Source: three-view drawing plus pictorial views. Frame: mm from the lowest corner of the part. A direction names the side the tool comes from. Coordinates: 2 decimals unless noted, no trailing zeros. Order: outer loops, then holes, each group sorted by start corner. A loop starts at its lowest first (then second) coordinate and runs counter-clockwise, first axis right, second up. Notation, with made-up numbers: (-2.5, 27.5) - (9.5, 27.5) arc R9 cw to (9.5, 31.5) - close; hole circle Ø4 at (-1, 20). An arc over 180 degrees is marked (long way). One line per question, with ' | ' between items.
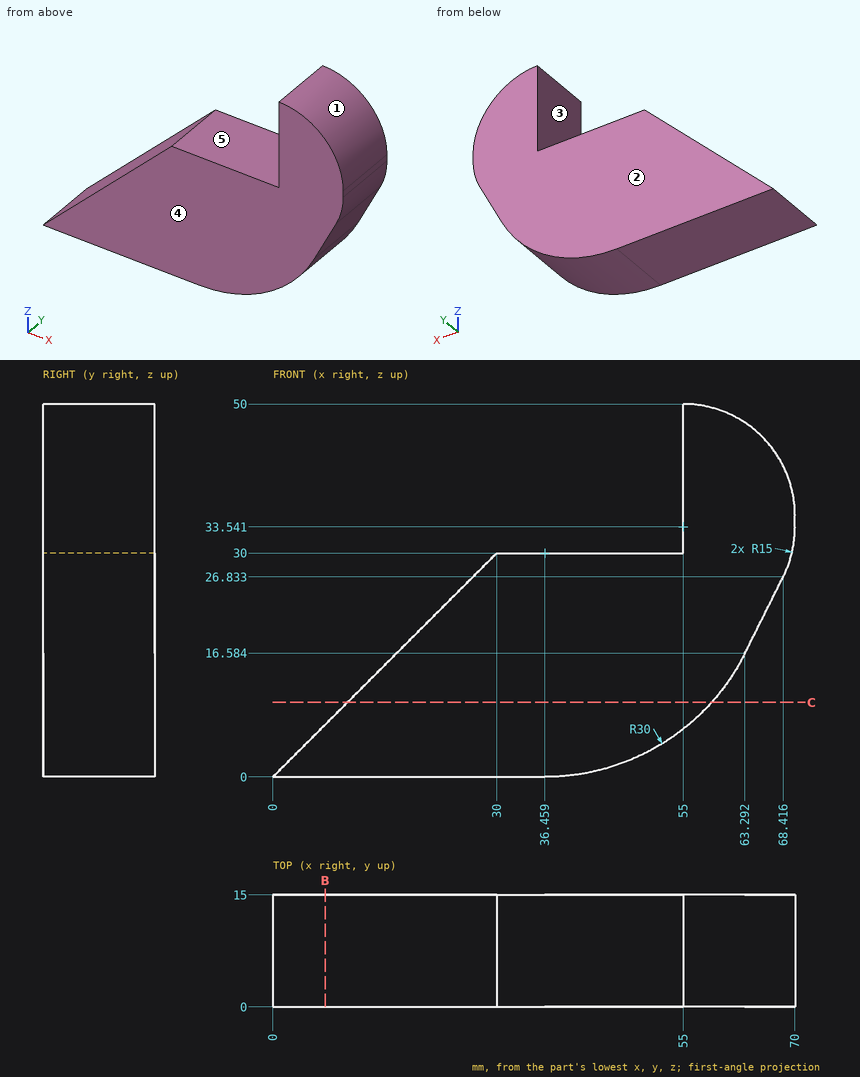
(1) Material intervals for L1, parallel to Z at x = 32, y = 11; L2, parallel to X at y = 4.75, z = 47.5; L3, parallel to X at y = 3, z = 28, sorted ascending. Write a range as from..to.
Taken from the geometry:
L1: z = 0..30 | L2: x = 55..63.29 | L3: x = 28..68.94
(2) Pin query (flat end, axial travel): P1, Ø2, axis at x = 57.5, y = 3.5, coming from the -Z side (1 decimal); P2, Ø8, axis at x = 21.5, y = 4.5, coming from the +Z side; P3, Ø1.5, axis at y = 5, z = 37, coming from the -X side. Return the tip coordinate at first contact, or that it passes through.
Taken from the geometry:
P1: stops at z = 7.7 | P2: stops at z = 25.5 | P3: stops at x = 55
(3) Set-up query: the marked faces 4 and 5. Return all of +Z, -Z, +X, -X, +Y, -Y with unobstructed straight access to the full face (end or side cutting, diameter ignored); none if empty.
Taken from the geometry:
face 4: +Z, -Z, +X, -X, -Y | face 5: +Z, -X, +Y, -Y
(4) Pull-direction query (X, two-part tool) for the marked faces 1, 2 and 3; classes: pulls with the +X half, pulls with the -X half, needs draft (parallel to the pull), parting line crosses it, or undercut.
Taken from the geometry:
face 1: pulls with the +X half | face 2: needs draft | face 3: pulls with the -X half
(5) Cut plane C-C (z = 10). Return the cut outline in (x, y).
Taken from the geometry:
outline: (10, 0) - (58.82, 0) - (58.82, 15) - (10, 15) - close
(6) Cut plane B-B (x = 7). Return the cut outline in (y, z), and give its area (3 significant figures).
Taken from the geometry:
outline: (0, 0) - (15, 0) - (15, 7) - (0, 7) - close | area: 105 mm²
